Design review of the part shown in the three views and the two pictorial views. Dimensions are in mm from the part's minimum x, y and z. A direction names the side the tool comes from. Coordinates: 2 decimals unless noted, no trailing zeros. Loops run counter-clockwise (first coordinate to the right, second up) from the corner with the lowest first, then second, coordinate; pieces in that order, holes last. Notation, with made-up numbers: (-4.75, 70.5) -> (5.25, 70.5) arc R21 ccw to (5.25, 84.5) -> close; hole circle Ø8 at (68, -23). An arc over 180 degrees is marked (long way). One line per item, written item: value.
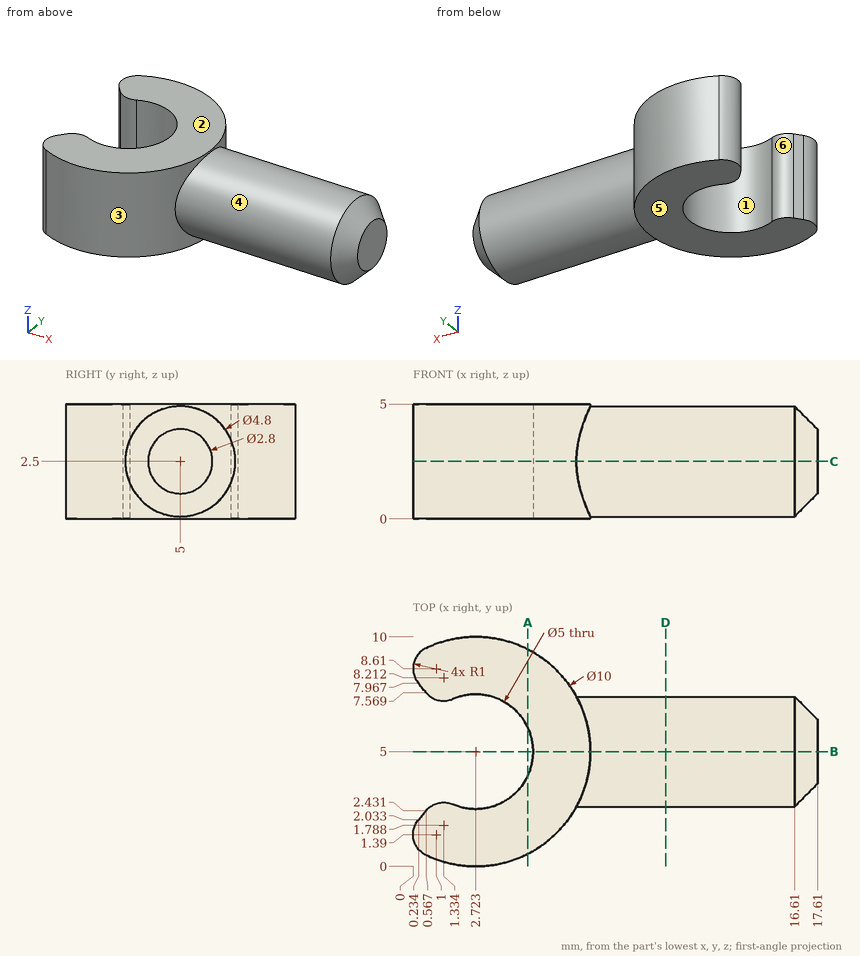
1. To check wall thickness, follow probe 1 along Y at (x, z) = (3.5, 3.6) (1 decimal); probe 2 along Y at (x, z) = (4.75, 1) (1 decimal); probe 3 along X at (y, z) = (8.75, 3.1). State the ranges of each line that lie inside material, in increasing order. Write a range as from..to.
Return value:
probe 1: y = 0.1..2.6, 7.4..9.9
probe 2: y = 0.4..3.5, 6.5..9.6
probe 3: x = 0.01..6.03
2. Take a section at A-A, the plane x = 5. Give the boundary of the cut face in (y, z).
Return value:
outline: (0.55, 0) -> (3.97, 0) -> (3.97, 5) -> (0.55, 5) -> close; (6.03, 0) -> (9.45, 0) -> (9.45, 5) -> (6.03, 5) -> close
3. For the marked faces 4, 5 and 6, list the 3-axis set-ups (+Z, -Z, +X, -X, +Y, -Y) from which the entire face can be reached by the end or side of a thin tool; tool diameter is ignored.
Return value:
face 4: +X
face 5: -Z, +X, -X, +Y, -Y
face 6: +Z, -Z
4. Insertion check: pin 1 Ø6 at (x, y) = (2.72, 5) entering from +Z; pin 2 Ø1 at (x, z) = (4, 3.5) entering from -Y. Each pin has a flat end and moves straight along its axis. Give the tip position at first contact, or say it passes through.
Return value:
pin 1: stops at z = 5
pin 2: stops at y = 0.06
5. Take a section at D-D, the plane x = 11. Give the boundary of the cut face in (y, z).
Return value:
outline: circle Ø4.8 at (5, 2.5)
6. Take a section at B-B, the plane y = 5. Give the boundary of the cut face in (x, z).
Return value:
outline: (5.22, 0) -> (7.72, 0) -> (7.72, 0.1) -> (16.61, 0.1) -> (17.61, 1.1) -> (17.61, 3.9) -> (16.61, 4.9) -> (7.72, 4.9) -> (7.72, 5) -> (5.22, 5) -> close
7. The part is to be moulded in two halves that separate along Y. For the marked faces 1, 2 and 3, say which applies: pulls with the +Y half, pulls with the -Y half, needs draft (parallel to the pull), parting line crosses it, or undercut.
Return value:
face 1: undercut
face 2: needs draft
face 3: parting line crosses it
8. Take a section at C-C, the plane z = 2.5. Give the boundary of the cut face in (x, y) (1 decimal).
Return value:
outline: (0.2, 2) arc R1 ccw to (0.6, 0.5) arc R5 ccw to (7.1, 2.6) -> (16.6, 2.6) -> (17.6, 3.6) -> (17.6, 6.4) -> (16.6, 7.4) -> (7.1, 7.4) arc R5 ccw to (0.6, 9.5) arc R1 ccw to (0.2, 8) -> (0.6, 7.6) arc R1 ccw to (1.7, 7.3) arc R2.5 cw (long way) to (1.7, 2.7) arc R1 ccw to (0.6, 2.4) -> close
